The model under review builds one solid part; all positions refer to its coordinate system, in mm. A direction names the side the tool comes from. Give positions to 0.01 mm unless a question says otherwise; leave off trailing zeros. Order: outer loops, then holes, each group sorted by start corner. A loop starts at its lowest first (then second) coordinate and runs counter-clockwise, first axis right, second up. Notation, with made-up numbers: (-14, -10.5) -> (24, -10.5) arc R19 cw to (24, 21.5) -> close; hole circle Ø9 at (52.5, 1.5). An arc over 180 degrees is marked (long way). Use one line per item in the form item = value.
```python
from build123d import *

# Parameters (mm, degrees)
SKETCH_W     = 23.20948
SKETCH_H     = 20.1
PAD_DEPTH    = 20
PAD001_DEPTH = 20
POCKET_DEPTH = 37.1


with BuildPart() as part:
    # Sketch → Pad (new body)
    with BuildSketch(Plane.XZ):
        Rectangle(SKETCH_W, SKETCH_H)
    extrude(amount=PAD_DEPTH)

    # Sketch001 (on DatumPlane) → Pad001 (join)
    with BuildSketch(Plane(origin=(0, 0, 10.05), x_dir=(-1, 0, 0), z_dir=(0, 0, 1))):
        Polygon((-5.744635, 19.95), (-11.48927, 10), (-5.744635, 0.05), (5.744635, 0.05), (11.48927, 10), (5.744635, 19.95), align=None)
    extrude(amount=PAD001_DEPTH)

    # Sketch002 (on Face13 of Pad001) → Pocket (cut)
    with BuildSketch(Plane(origin=(0, 0, 30.05), x_dir=(-1, 0, 0), z_dir=(0, 0, 1))):
        Polygon((3.781644, 16.55), (-3.781644, 16.55), (-7.563289, 10), (-3.781644, 3.45), (3.781644, 3.45), (7.563289, 10), align=None)
    extrude(amount=-POCKET_DEPTH, mode=Mode.SUBTRACT)


solid = part.part
```
1. Add section B-B on x = -1.5. Give the boundary of the cut face in (y, z).
Values:
outline = (-20, -10.05) -> (0, -10.05) -> (0, 10.05) -> (-0.05, 10.05) -> (-0.05, 30.05) -> (-3.45, 30.05) -> (-3.45, -7.05) -> (-16.55, -7.05) -> (-16.55, 30.05) -> (-19.95, 30.05) -> (-19.95, 10.05) -> (-20, 10.05) -> close
2. Tool access review of faces 1 (the face through (0, -20, 0)), 2 (the face through (8.657, -5.095, 19.91)), 3 (the face through (-8.657, -14.905, 19.91)), 4 (the face through (0, -0.05, 20)), 5 (the face through (0, -16.55, 12)): name each direction out of +Z, -Z, +X, -X, +Y, -Y from which nothing blocks a thin tool from reaching the whole face with its end or side.
Values:
face_1 = +Z, -Z, +X, -X, -Y
face_2 = +Z, +X, +Y
face_3 = +Z, -X, -Y
face_4 = +Z, +X, -X, +Y
face_5 = +Z
3. Add section A-A on z = 1.5. Give the boundary of the cut face in (x, y).
Values:
outline = (-11.6, -20) -> (11.6, -20) -> (11.6, 0) -> (-11.6, 0) -> close; hole (-7.56, -10) -> (-3.78, -16.55) -> (3.78, -16.55) -> (7.56, -10) -> (3.78, -3.45) -> (-3.78, -3.45) -> close
4. For pin 1 Ø1 at (x, z) = (-9, 18) entering from +Y; pin 2 Ø8 at (y, z) = (-13, 11.5) entering from -X; pin 3 Ø5.5 at (x, z) = (1, 20.5) entering from +Y; pin 4 Ø3.5 at (x, z) = (3, 18.5) entering from -Y, all flat-tipped, find the tip position at first contact; note any pin that passes through.
Values:
pin_1 = -4.82
pin_2 = -11.6
pin_3 = -0.05
pin_4 = -19.95
5. The part is to be moulded in two halves that separate along Y. For faces 6 (the face through (0, -3.45, 12)), 7 (the face through (-5.646, -6.679, 11.76)), 8 (the face through (-11.605, -10, 0)), 9 (the face through (-8.58, -4.96, 19.91)), say which applies: +Y half, -Y half, draft (parallel to the pull), parting line (faces both ways), or undercut.
Values:
face_6 = undercut
face_7 = undercut
face_8 = draft
face_9 = +Y half
6. Add section D-D on z = 28.5. Give the boundary of the cut face in (x, y), then the cut area to 3 significant figures.
Values:
outline = (-11.49, -10) -> (-5.74, -19.95) -> (5.74, -19.95) -> (11.49, -10) -> (5.74, -0.05) -> (-5.74, -0.05) -> close; hole (-7.56, -10) -> (-3.78, -16.55) -> (3.78, -16.55) -> (7.56, -10) -> (3.78, -3.45) -> (-3.78, -3.45) -> close
area = 194 mm^2
7. Add section C-C on y = -18.5. Give the boundary of the cut face in (x, z).
Values:
outline = (-11.6, -10.05) -> (11.6, -10.05) -> (11.6, 10.05) -> (6.58, 10.05) -> (6.58, 30.05) -> (-6.58, 30.05) -> (-6.58, 10.05) -> (-11.6, 10.05) -> close
8. For L1, parallel to Y at x = 2.75, z = 3.5; L2, parallel to Z at x = -3.25, y = -16.25; L3, parallel to Z at x = -8.75, y = -17, list the stretches that pass through material, from the lowest coordinate up.
Values:
L1 = -20 to -16.55, -3.45 to 0
L2 = -10.05 to -7.05
L3 = -10.05 to 10.05
